Autodesk Inventor part; units mm, degrees
ref_plane "YZ Plane" through (0, 0, 0) normal (1, 0, 0) x (0, 1, 0)
ref_plane "XZ Plane" through (0, 0, 0) normal (0, 1, 0) x (-1, 0, 0)
ref_plane "XY Plane" through (0, 0, 0) normal (0, 0, 1) x (1, 0, 0)
sketch "Sketch1" plane through (0, 0, 0) normal (1, 0, 0) x (0, 1, 0)
  arc A0 (-20.6375, 0) -> (20.6375, 0) centre (0, 0) ccw
  arc A1 (20.6375, 115.5112) -> (-20.6375, 115.5112) centre (0, 115.5112) ccw
  line L0 (-20.6375, 115.5112) -> (-20.6375, 0)
  line L1 (20.6375, 0) -> (20.6375, 115.5112)
  dimension "d0" = 115.5112
  dimension "d1" = 41.275
extrude "Plate1" add sketch "Sketch1" along normal blind 3.175
sketch "Sketch2" plane through (3.175, 0, 0) normal (1, 0, 0) x (0, 0, -1)
  point P0 (0, 0)
  point P1 (0, 0)
  point P2 (0, 0)
  point P3 (-115.5112, 0)
  dimension "d21" = 115.5112
hole "Hole1" at (3.175, 0, 0) at (3.175, 0, 115.5112) direction (-1, 0, 0) diameter 28.575 depth 3.175 tip angle 118
sketch "Sketch3" plane through (3.175, 0, 0) normal (1, 0, 0) x (0, 0, -1)
  circle A0 centre (0, 0) radius 15.5575 construction
  point P0 (-18.288, 0)
  point P1 (-115.5112, 0)
  point P2 (-97.2232, 0)
  dimension "d10" = 31.115
  dimension "d13" = 18.288
  dimension "d22" = 115.5112
  dimension "d23" = 18.288
hole "Hole2" at (3.175, 0, 18.288) at (3.175, 0, 97.2232) direction (-1, 0, 0) diameter 3.9624 depth 13.6144 tip angle 118
equation "\"d8\" = Thickness"
equation "\"d2\" = Thickness"
equation "\"BendRadius\" = Thickness"
equation "\"BendReliefWidth\" = Thickness"
equation "\"BendReliefDepth\" = 0.5 * Thickness"
equation "\"CornerReliefSize\" = 4 * Thickness"
equation "\"MinimumRemnant\" = 2 * Thickness"
equation "\"TransitionRadius\" = BendRadius"
equation "\"JacobiRadiusSize\" = BendRadius"
equation "\"GapSize\" = Thickness"
properties part number "PLATE,KICKER,MOTOR,SUPPORT" material "Polycarbonate, Clear"
Geometry check sheet. Reference: the model listing, model coordinates, mm. Round coordinates to 2 decimals unless told otherwise and drop trailing zeros. Loops run counter-clockwise (first coordinate to the right, second up) from the corner with the lowest first, then second, coordinate; pieces in that order, holes last. Notation, with made-up numbers: (4, 3) - (52, 3) arc R32 cw to (52, 38) - close; hole circle Ø3 at (-25, 83). An arc over 180 degrees is marked (long way). Write item = value, one per line. Start each with the question number.
1. Mould release check, pull along Z, two halves, no side actions. Record for faces 1 (the face through (0, 0, 59)), 2 (the face through (1.565, -0.454, 136.144)), 3 (the face through (1.565, -0.087, 20.267)): released by +Z, released by -Z, zero draft, split by the parting line, or undercut.
2. Thickness scan on line 1 (Z direction, x = 1.85, y = 0); line 2 (Z direction, x = 2.2, y = 9); line 3 (Y direction, x = 1.55, z = 0). Record the ranges inside material, lowest first.
3. Section check B-B on z = 110.5. Enter the section's corners in (x, y) (1 decimal), then the cut area to 3 significant figures.
4. Section check D-D on y = 6.5. Enter the section's corners in (x, z) (3 decimals).
5. Section check A-A on y = 0. Enter the section's corners in (x, z) (1 decimal).
6. Section check C-C on x = 0.5. Enter the section's corners in (y, z) (1 decimal), then the cut area to 3 significant figures.
Working result:
q1.face_1 = zero draft
q1.face_2 = released by +Z
q1.face_3 = undercut
q2.line_1 = -20.64 to -14.29, 14.29 to 16.31, 20.27 to 95.24, 99.2 to 101.22, 129.8 to 136.15
q2.line_2 = -18.57 to -11.1, 11.1 to 104.41, 126.61 to 134.08
q2.line_3 = -20.64 to -14.29, 14.29 to 20.64
q3.outline = (0, -20.6) - (3.2, -20.6) - (3.2, -13.4) - (0, -13.4) - close; (0, 13.4) - (3.2, 13.4) - (3.2, 20.6) - (0, 20.6) - close
q3.area = 46.1 mm^2
q4.outline = (0, -19.587) - (3.175, -19.587) - (3.175, -12.723) - (0, -12.723) - close; (0, 12.723) - (3.175, 12.723) - (3.175, 102.788) - (0, 102.788) - close; (0, 128.235) - (3.175, 128.235) - (3.175, 135.098) - (0, 135.098) - close
q5.outline = (0, -20.6) - (3.2, -20.6) - (3.2, -14.3) - (0, -14.3) - close; (0, 14.3) - (3.2, 14.3) - (3.2, 16.3) - (0, 16.3) - close; (0, 20.3) - (3.2, 20.3) - (3.2, 95.2) - (0, 95.2) - close; (0, 99.2) - (3.2, 99.2) - (3.2, 101.2) - (0, 101.2) - close; (0, 129.8) - (3.2, 129.8) - (3.2, 136.1) - (0, 136.1) - close
q6.outline = (-20.6, 0) arc R20.6 ccw to (20.6, 0) - (20.6, 115.5) arc R20.6 ccw to (-20.6, 115.5) - close; hole circle Ø28.6 at (0, 0); hole circle Ø28.6 at (0, 115.5); hole circle Ø4 at (0, 18.3); hole circle Ø4 at (0, 97.2)
q6.area = 4,800 mm^2
